Autodesk Inventor part; units mm, degrees
ref_plane "YZ Plane" through (0, 0, 0) normal (1, 0, 0) x (0, 1, 0)
ref_plane "XZ Plane" through (0, 0, 0) normal (0, 1, 0) x (-1, 0, 0)
ref_plane "XY Plane" through (0, 0, 0) normal (0, 0, 1) x (1, 0, 0)
sketch "Sketch1" plane through (0, 0, 0) normal (0, 0, 1) x (1, 0, 0)
  line L0 (0, 0) -> (0, 30.3704) construction
  line L1 (0, 0) -> (7.18, 0)
  line L2 (7.18, 0) -> (7.18, 4.46)
  arc A0 (0, 2.4704) -> (0, 30.3704) centre (0, 16.4204) ccw
  line L3 (13.5038, 19.9204) -> (17.75, 19.9204)
  arc A1 (17.75, 12.9204) -> (17.75, 19.9204) centre (17.75, 16.4204) ccw
  line L4 (17.75, 12.9204) -> (13.5038, 12.9204)
  circle A2 centre (17.75, 16.4204) radius 2
  line L5 (0, 0) -> (-7.18, 0)
  line L6 (-7.18, 0) -> (-7.18, 4.46)
  arc A3 (0, 30.3704) -> (0, 2.4704) centre (0, 16.4204) ccw
  line L7 (-13.5038, 19.9204) -> (-17.75, 19.9204)
  arc A4 (-17.75, 19.9204) -> (-17.75, 12.9204) centre (-17.75, 16.4204) ccw
  line L8 (-17.75, 12.9204) -> (-13.5038, 12.9204)
  circle A5 centre (-17.75, 16.4204) radius 2
  circle A6 centre (0, 24.3704) radius 4.61
  circle A7 centre (0, 24.3704) radius 2.5
  line L9 (2.0541, 25.7954) -> (-2.0541, 25.7954)
  line L10 (2.0541, 22.9454) -> (-2.0541, 22.9454)
  dimension "d0" = 13.95
  dimension "d1" = 7.18
  dimension "d2" = 4.46
  dimension "d3" = 3.5
  dimension "d4" = 4
  dimension "d11" = 9.22
  dimension "d12" = 5
  dimension "d13" = 2.85
  dimension "d26" = 35.5
  dimension "d27" = 6
extrude "Extrusion1" add sketch "Sketch1" along normal blind 19.2 contours A0 A3 | A6 | A7 L10 L9 | L9 A7 | A7 L10
extrude "Extrusion2" add sketch "Sketch1" along normal blind 0.79 contours A0 L3 A1 L4 | L8 A4 L7 A3
extrude "Extrusion3" add sketch "Sketch1" along normal blind 16.5 contours L5 L6 A3 A0 L2 L1
extrude "Extrusion4" add sketch "Sketch1" against normal blind 1.75 contours A6
extrude "Extrusion5" add sketch "Sketch1" against normal blind 3.78 contours L9 A7 | A7 L10
extrude "Extrusion6" add sketch "Sketch1" against normal blind 9.73 contours A7 L10 L9
fillet "Fillet1" radius 1.2 6 edges at (7.18, 28.3807, 19.2) (7.18, 0, 8.25) (0, 0, 16.5) (-7.18, 0, 8.25) (-7.18, 2.23, 16.5) (7.18, 2.23, 16.5)
sketch "Sketch2" plane through (-5.98, 0, 0) normal (0, -1, 0) x (1, 0, 0)
  line L0 (8.98, 2.56) -> (2.98, 2.56) construction
  line L1 (8.98, 2) -> (2.98, 2)
  line L2 (2.98, 3.12) -> (8.98, 3.12)
  arc A0 (8.98, 2) -> (8.98, 3.12) centre (8.98, 2.56) ccw
  arc A1 (2.98, 3.12) -> (2.98, 2) centre (2.98, 2.56) ccw
  line L3 (0, 0) -> (11.96, 0)
  point P0 (5.98, 0)
  point P1 (5.98, 2.56)
  point P2 (5.98, 0)
  dimension "d21" = 2
  dimension "d22" = 1.12
  dimension "d23" = 6
extrude "Extrusion7" cut sketch "Sketch2" against normal blind 2
properties part number "STEPPER MOTOR"
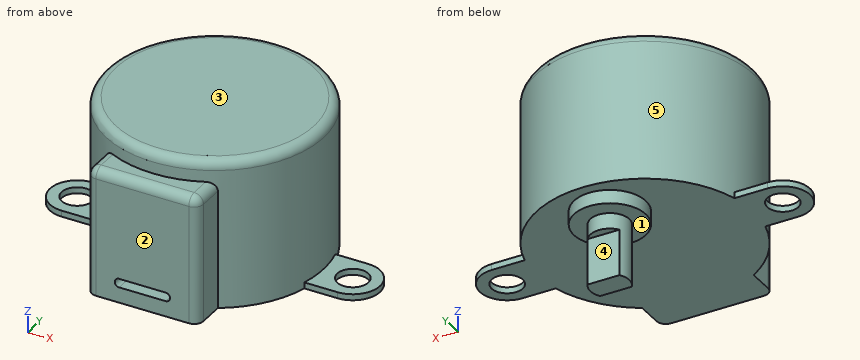
Geometry: final body of the model. Coordinates: model frame, mm. Face numbers are marked on the shaded views. A direction names the side the tool comes from. Give positions to 0.01 mm unless a question says otherwise; leave off trailing zeros. Write each loop counter-clockwise with the first axis right and the second up, starting at its lowest first coordinate (ties: lowest second). Pieces come first, ordered by that corner, then holes.
(1) Cut plane B-B, the plane z = 10. Return loops of the section in (x, y).
(2) Ray query, line 1 (Y direction, x = 17.75, z = 0.25); line 2 (Z direction, x = 3, y = 22); line 3 (X direction, y = 17, z = 8.5). Return the intervals inside material, ascending.
(3) First-contact query: P1, Ø4, axis at x = -11, z = 9.5, coming from the +Y side; P2, Ø0.8, axis at x = 3, y = 2, coming from the +Z side; P3, Ø4, axis at y = 22.5, z = 0, coming from the +X side; P4, Ø2.5, axis at x = -17.75, y = 16.42, coming from the -Z side. Flat tips, straight axial feed; report the tip coordinate or a pass-through.
(4) Cut plane D-D, the plane z = -2.75. Return loops of the section in (x, y).
(5) Cut plane A-A, the plane x = 0. Return loops of the section in (y, z).
(6) Cut plane C-C, the plane z = 2.56. Return loops of the section in (x, y).
(7) Access query for the marked faces 1, 2, 3, 4 and 5. Directions: +Z, -Z, +X, -X, +Y, -Y. A direction counts if a zero-diameter tool reaches every point of the face in a straight line with its end or side. Return the directions, or none.
Values follow:
1. outline: (-7.18, 1.2) arc R1.2 ccw to (-5.98, 0) - (5.98, 0) arc R1.2 ccw to (7.18, 1.2) - (7.18, 4.46) arc R13.95 ccw (long way) to (-7.18, 4.46) - close
2. line 1: y = 12.92 to 14.42, 18.42 to 19.92
2. line 2: z = -1.75 to 19.2
2. line 3: x = -13.94 to 13.94
3. P1: stops at y = 27.08
3. P2: stops at z = 16.5
3. P3: stops at x = 13.34
3. P4: passes through
4. outline: circle Ø5 at (0, 24.37)
5. outline: (0, 0) - (19.76, 0) - (19.76, -1.75) - (21.87, -1.75) - (21.87, -3.78) - (22.95, -3.78) - (22.95, -9.73) - (25.8, -9.73) - (25.8, -3.78) - (26.87, -3.78) - (26.87, -1.75) - (28.98, -1.75) - (28.98, 0) - (30.37, 0) - (30.37, 18) arc R1.2 ccw to (29.17, 19.2) - (3.67, 19.2) arc R1.2 ccw to (2.47, 18) - (2.47, 16.5) - (1.2, 16.5) arc R1.2 ccw to (0, 15.3) - (0, 3.12) - (2, 3.12) - (2, 2) - (0, 2) - close
6. outline: (-7.18, 1.2) arc R1.2 ccw to (-5.98, 0) - (-3.56, 0) - (-3.56, 2) - (3.56, 2) - (3.56, 0) - (5.98, 0) arc R1.2 ccw to (7.18, 1.2) - (7.18, 4.46) arc R13.95 ccw (long way) to (-7.18, 4.46) - close
7. face 1: -Z
7. face 2: +Z, -Z, +X, -X, -Y
7. face 3: +Z, +X, -X, +Y, -Y
7. face 4: -Z, +X, -X, +Y
7. face 5: +Z
